Design review of the part built by this model. Coordinates are the model's own, in mm. A direction names the side the tool comes from. Give positions to 0.01 mm unless a question says otherwise; leave off trailing zeros. Loops run counter-clockwise (first coordinate to the right, second up) from the corner with the lowest first, then second, coordinate; pieces in that order, holes last. Notation, with made-up numbers: M 62,31 L 111,31 A18 ccw 111,51 Z; hole C -20,18.5 d7. An arc over 180 degrees is marked long. Use one line per item in the form item = value. Start each with the question number.
from build123d import *

# Parameters (mm, degrees)
BOSS_EXTRU_1_DEPTH      = 10
ESQUISSE5_R             = 1.036050106
ENL_V_MAT_EXTRU_2_DEPTH = 42


with BuildPart() as part:
    # Esquisse2 → Boss.-Extru.1 (new body)
    with BuildSketch(Plane(origin=(0, 0, 0), x_dir=(1, 0, 0), z_dir=(0, 1, 0))):
        with BuildLine():
            Line((24.963471106, -20), (30.003471106, -20))
            Line((30.003471106, -20), (30.003471106, -19))
            Line((30.003471106, -19), (24.963471106, -19))
            ThreePointArc((24.963471106, -19), (22.092040168, -17.073276579), (20.970186635, -13.802370983))
            Line((20.970186635, -13.802370983), (20.970186635, 1.118602927))
            ThreePointArc((20.970186635, 1.118602927), (0, 21), (-20.970186635, 1.118602927))
            Line((-20.970186635, 1.118602927), (-20.970186635, -13.802370983))
            ThreePointArc((-20.970186635, -13.802370983), (-22.092040168, -17.073276579), (-24.963471106, -19))
            Line((-24.963471106, -19), (-30.003471106, -19))
            Line((-30.003471106, -19), (-30.003471106, -20))
            Line((-30.003471106, -20), (-24.963471106, -20))
            ThreePointArc((-24.963471106, -20), (-21.402232401, -17.765722993), (-20, -13.802370983))
            Line((-20, -13.802370983), (-20, 0))
            ThreePointArc((-20, 0), (0, 20), (20, 0))
            Line((20, 0), (20, -13.802370983))
            ThreePointArc((20, -13.802370983), (21.402232401, -17.765722993), (24.963471106, -20))
        make_face()
    extrude(amount=BOSS_EXTRU_1_DEPTH)

    # Esquisse5 → Enlèv. mat.-Extru.2 (cut, through all)
    with BuildSketch(Plane.XY.offset(20)):
        with Locations((-27.503471106, 7.5)):
            Circle(ESQUISSE5_R)
        with Locations((-27.503471106, 2.5)):
            Circle(ESQUISSE5_R)
        with Locations((27.503471106, 2.5)):
            Circle(ESQUISSE5_R)
        with Locations((27.503471106, 7.5)):
            Circle(ESQUISSE5_R)
    extrude(amount=-ENL_V_MAT_EXTRU_2_DEPTH, mode=Mode.SUBTRACT)


solid = part.part
Q1. Take a section at B-B on z = 3. Give the boundary of the cut face in (x, y).
Q2. Wall thickness on probe 1 along X at (y, z) = (0.75, 8); probe 2 along X at (y, z) = (5.5, -12.5); probe 3 along Z at (x, y) = (7, 6.25) (3 decimals): over which ranges is each line inside the solid? List them lowest first.
Q3. Take a section at A-A on y = 7.5. Give the boundary of the cut face in (x, z).
Q4. The part is to be moulded in two halves that separate along Y. For faces 1 (the cylindrical face through (26.47, 7.55, 19.51)), 2 (the flat face through (-18, 10, -10)), 3 (the flat face through (-27, 5, 19)), say which applies: pulls with the +Y half, pulls with the -Y half, needs draft (parallel to the pull), parting line crosses it, or undercut.
Q5. Take a section at C-C on x = 0. Give the boundary of the cut face in (y, z), plus the area to 3 significant figures.
Q6. For faces 4 (the flat face through (20.97, 5, 6)), 5 (the flat face through (-20.97, 5, 6)), 6 (the cylindrical face through (-28.54, 7.55, 19.51)), 7 (the flat face through (20, 5, 7)), list the 3-axis set-ups (+Z, -Z, +X, -X, +Y, -Y) from which the entire face can be reached by the end or side of a thin tool; tool diameter is ignored.
Q7. Take a section at D-D on z = -12.5. Give the boundary of the cut face in (x, y).
Q8. Clearance check with flat-ended pins moving along their axes: pin 1 Ø1.5 at (x, y) = (26.5, 6) entering from -Z; pin 2 Ø1.5 at (y, z) = (4.5, -0.5) entering from +X; pin 3 Ø4 at (x, y) = (-11, 2) entering from +Z. State where each tip first meets the part, or that it passes through.
Response values:
q1.outline = M -20.97,0 L -20,0 L -20,10 L -20.97,10 Z; M 20,0 L 20.97,0 L 20.97,10 L 20,10 Z
q2.probe_1 = -20.97 to -20, 20 to 20.97
q2.probe_2 = -16.87 to -15.61, 15.61 to 16.87
q2.probe_3 = -19.799 to -18.735
q3.outline = M -30,19 L -28.54,19 L -28.54,20 L -30,20 Z; M -26.47,19 L -24.96,19 A5.42 cw -20.97,13.8 L -20.97,-1.12 A21 ccw 20.97,-1.12 L 20.97,13.8 A5.42 cw 24.96,19 L 26.47,19 L 26.47,20 L 24.96,20 A6.39 ccw 20,13.8 L 20,0 A20 cw -20,0 L -20,13.8 A6.39 ccw -24.96,20 L -26.47,20 Z; M 28.54,19 L 30,19 L 30,20 L 28.54,20 Z
q4.face_1 = undercut
q4.face_2 = pulls with the +Y half
q4.face_3 = needs draft
q5.outline = M 0,-21 L 10,-21 L 10,-20 L 0,-20 Z
q5.area = 10.0 mm^2
q6.face_4 = -Z, +X, +Y, -Y
q6.face_5 = -Z, -X, +Y, -Y
q6.face_6 = +Z, -Z
q6.face_7 = +Z, +Y, -Y
q7.outline = M -16.87,0 L -15.61,0 L -15.61,10 L -16.87,10 Z; M 15.61,0 L 16.87,0 L 16.87,10 L 15.61,10 Z
q8.pin_1 = 19
q8.pin_2 = 20.97
q8.pin_3 = -15.2
